from build123d import *

# Parameters (mm, degrees)
SKETCH1_R                                           = 40.3225
BOSS_EXTRUDE1_DEPTH                                 = 9.525
SKETCH2_R                                           = 42.545
BOSS_EXTRUDE2_DEPTH                                 = 6.35
SKETCH3_R                                           = 57.15
BOSS_EXTRUDE3_DEPTH                                 = 6.35
FILLET2_R                                           = 2.54
CSK_FOR_1_4_FLAT_HEAD_MACHINE_SCREW_100_D           = 6.7564
CSK_FOR_1_4_FLAT_HEAD_MACHINE_SCREW_100_CSINK_D     = 12.8778
CSK_FOR_1_4_FLAT_HEAD_MACHINE_SCREW_100_CSINK_ANGLE = 100


with BuildPart() as part:
    # Sketch1 → Boss-Extrude1 (new body)
    with BuildSketch(Plane(origin=(0, 0, 0), x_dir=(1, 0, 0), z_dir=(0, 1, 0))):
        with Locations(Location((0, 0, 0), (0, 0, 90))):
            Circle(SKETCH1_R)
    extrude(amount=BOSS_EXTRUDE1_DEPTH)

    # Sketch2 → Boss-Extrude2 (add)
    with BuildSketch(Plane.XZ):
        with Locations(Location((0, 0, 0), (0, 0, 270))):
            Circle(SKETCH2_R)
    extrude(amount=BOSS_EXTRUDE2_DEPTH)

    # Sketch3 → Boss-Extrude3 (add)
    with BuildSketch(Plane.XZ.offset(6.35)):
        with Locations(Location((0, 0, 0), (0, 0, 270))):
            Circle(SKETCH3_R)
    extrude(amount=BOSS_EXTRUDE3_DEPTH)

    # Fillet2
    fillet2_edges = [part.edges().sort_by_distance(p)[0] for p in [
        (0, -6.35, 57.15),
    ]]
    fillet(fillet2_edges, radius=FILLET2_R)

    # CSK for 1/4 Flat Head Machine Screw (100)1 (through all)
    with Locations(Plane(origin=(0, -12.7, 0), x_dir=(0, 0, -1), z_dir=(0, -1, 0))):
        with Locations((0, 0)):
            CounterSinkHole(CSK_FOR_1_4_FLAT_HEAD_MACHINE_SCREW_100_D / 2, CSK_FOR_1_4_FLAT_HEAD_MACHINE_SCREW_100_CSINK_D / 2, counter_sink_angle=CSK_FOR_1_4_FLAT_HEAD_MACHINE_SCREW_100_CSINK_ANGLE)


solid = part.part
Design review of the part built by this model. Coordinates are the model's own, in mm. A direction names the side the tool comes from. Round coordinates to 2 decimals unless told otherwise and drop trailing zeros. Loops run counter-clockwise (first coordinate to the right, second up) from the corner with the lowest first, then second, coordinate; pieces in that order, holes last. Notation, with made-up numbers: M 21,-30 L 55,-30 A18 ccw 55,0 Z; hole C -3,11 d6. An arc over 180 degrees is marked long. Answer as a JSON object with one key per item and string values.
Item 1: We need section D-D on y = -4. Give the boundary of the cut face in (x, z) (3 decimals), and give its area (3 significant figures).
Answer sheet:
{"outline": "C 0,0 d85.09; hole C 0,0 d6.756", "area": "5,650 mm^2"}
Item 2: We need section C-C on y = 7.25. Give the boundary of the cut face in (x, z) (1 decimal).
Answer sheet:
{"outline": "C 0,0 d80.6; hole C 0,0 d6.8"}
Item 3: Machinability: for faces 4 (the cylindrical face through (-41.533, -3.131, 9.223)), 5 (the conical face through (-2.15, -10.26, -2.8)), which of the approach directions +Z, -Z, +X, -X, +Y, -Y give a long, thin tool a straight path to every point of the face, cutting with its end or side? Answer none if there is none.
Answer sheet:
{"face 4": "+Y", "face 5": "-Y"}
Item 4: Clearance check with flat-ended pins moving along their axes: P1, Ø4, axis at x = -13, y = -9, coming from the -Z side; P2, Ø8, axis at x = -15.5, y = 6.5, coming from the -Z side; P3, Ø11, axis at x = 0, z = 0, coming from the -Y side. State where each tip first meets the part, or that it passes through.
Answer sheet:
{"P1": "stops at z = -56.08", "P2": "stops at z = -38.65", "P3": "stops at y = -11.91"}
Item 5: Wall thickness on L1, parallel to X at y = 3.25, z = 0; L2, parallel to X at y = -4, z = 0 (3 decimals); L3, parallel to Y at x = 13.5, z = -44.5: over which ranges is each line inside the solid? List them lowest first. Write a range as from..to.
Answer sheet:
{"L1": "x = -40.32..-3.38, 3.38..40.32", "L2": "x = -42.545..-3.378, 3.378..42.545", "L3": "y = -12.7..-6.35"}
Item 6: The part is to be moulded in two halves that separate along Z. For faces 1 (the flat face through (-38, 0, -16)), 2 (the cylindrical face through (-2.056, -0.166, -2.681)), 3 (the cylindrical face through (-34, 4.7, -21.68)), say which applies: pulls with the +Z half, pulls with the -Z half, needs draft (parallel to the pull), parting line crosses it, or undercut.
Answer sheet:
{"face 1": "needs draft", "face 2": "undercut", "face 3": "parting line crosses it"}
